For this review, use the dimensioned drawing (mm, ordinates from the lowest corner) and the shaded views. Coordinates: 2 decimals unless noted, no trailing zeros. Order: outer loops, then holes, each group sorted by start corner. A loop starts at its lowest first (then second) coordinate and runs counter-clockwise, first axis right, second up. Notation, with made-up numbers: M 89.5,6 L 106.5,6 A12 cw 106.5,11 Z; hole C -33.75,7.25 d7. An arc over 180 degrees is marked long. Answer in a Markdown table with one row per item.
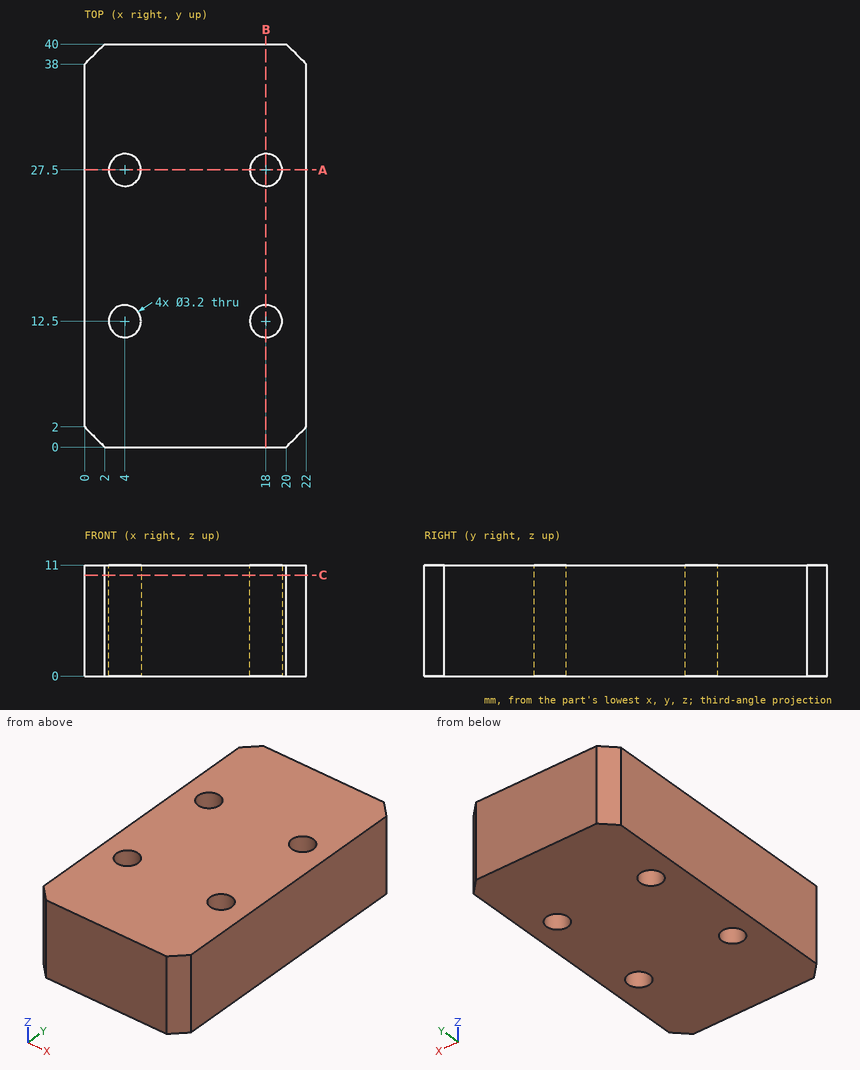
(1) Insertion check: pin 1 Ø2.5 at (x, y) = (18, 12.5) entering from -Z. The pin has a flat end and moves straight along its axis. Give the tip position at first contact, or say it passes through.
Return value:
| item | result |
|---|---|
| pin 1 | passes through |
(2) Add section C-C, the plane z = 10. Give the boundary of the cut face in (x, y), and give its area (3 significant figures).
Return value:
| item | result |
|---|---|
| outline | M 0,2 L 2,0 L 20,0 L 22,2 L 22,38 L 20,40 L 2,40 L 0,38 Z; hole C 4,12.5 d3.2; hole C 4,27.5 d3.2; hole C 18,12.5 d3.2; hole C 18,27.5 d3.2 |
| area | 840 mm2 |
(3) Add section A-A, the plane y = 27.5. Give the boundary of the cut face in (x, z).
Return value:
| item | result |
|---|---|
| outline | M 0,0 L 2.4,0 L 2.4,11 L 0,11 Z; M 5.6,0 L 16.4,0 L 16.4,11 L 5.6,11 Z; M 19.6,0 L 22,0 L 22,11 L 19.6,11 Z |
(4) For line 1 along Y through (x, z) = (18, 7.75); line 2 along Y through (x, z) = (2.75, 3.5); line 3 along X through (y, z) = (38.5, 6.75), list the stretches that pass through material, from the lowest coordinate up. Write a range as from..to.
Return value:
| item | result |
|---|---|
| line 1 | y = 0..10.9, 14.1..25.9, 29.1..40 |
| line 2 | y = 0..11.5, 13.5..26.5, 28.5..40 |
| line 3 | x = 0.5..21.5 |
(5) Add section B-B, the plane x = 18. Give the boundary of the cut face in (y, z), and give its area (3 significant figures).
Return value:
| item | result |
|---|---|
| outline | M 0,0 L 10.9,0 L 10.9,11 L 0,11 Z; M 14.1,0 L 25.9,0 L 25.9,11 L 14.1,11 Z; M 29.1,0 L 40,0 L 40,11 L 29.1,11 Z |
| area | 370 mm2 |
